```python
from build123d import *

# Parameters (mm, degrees)
F0_R     = 6.35
F1_DEPTH = 60
F3_DEPTH = 12
F4_R     = 1.5
F5_DEPTH = 25


with BuildPart() as f1:
    # F0 (on Front) → F1 (new body)
    with BuildSketch(Plane.XZ):
        Circle(F0_R)
    extrude(amount=-F1_DEPTH)

    # F2 (on face) → F3 (cut)
    with BuildSketch(Plane(origin=(0, 60, 0), x_dir=(-1, 0, 0), z_dir=(0, 1, 0))):
        Polygon((-6.955139, 0), (-4.5, -7.185974), (-4.5, 7.369376), align=None)
        Polygon((4.5, 7.369376), (4.5, -7.185974), (6.955139, 0), align=None)
    extrude(amount=-F3_DEPTH, mode=Mode.SUBTRACT)

    # F4 (on face) → F5 (cut)
    with BuildSketch(Plane.YZ.offset(4.5)):
        with Locations((56, 0)):
            Circle(F4_R)
    extrude(amount=-F5_DEPTH, mode=Mode.SUBTRACT)


solid = f1.part
```
Could you check a few things on this model? Use its own coordinates, in mm. A direction names the side the tool comes from. Round coordinates to 2 decimals unless told otherwise and drop trailing zeros. Loops run counter-clockwise (first coordinate to the right, second up) from the corner with the lowest first, then second, coordinate; pieces in that order, holes last. Notation, with made-up numbers: M 31,-25 L 88,-25 A19 cw 88,-21 Z; hole C -8.75,63.25 d7. An arc over 180 degrees is marked long. Answer as CSV lines item,"result".
1) We'd pull the mould along Z, two halves only. Please class faces 4 (the cylindrical face through (6.057, 29.58, 1.907)), 5 (the flat face through (4.5, 54, 0)), 6 (the cylindrical face through (0.06, 57.43, 0.45)): released by +Z, released by -Z, zero draft, split by the parting line, or undercut.
From the geometry:
face 4,"split by the parting line"
face 5,"zero draft"
face 6,"undercut"
2) Imagine slicing it at D-D on y = 24. List the corners of the cut face in (x, z) for me.
From the geometry:
outline,"C 0,0 d12.7"
3) Imagine slicing it at A-A on z = 0. List the corners of the cut face in (x, y) for me, and give its area (3 significant figures).
From the geometry:
outline,"M -6.35,0 L 6.35,0 L 6.35,48 L 4.5,48 L 4.5,54.5 L -4.5,54.5 L -4.5,48 L -6.35,48 Z; M -4.5,57.5 L 4.5,57.5 L 4.5,60 L -4.5,60 Z"
area,"691 mm^2"
4) Which directions (+Z, -Z, +X, -X, +Y, -Y) give clear straight access to the entire face, cutting with the end or side of a thin tool? Please do faces 1 (the flat face through (5, 48, 0)), 2 (the flat face through (0, 0, 0)), 3 (the flat face through (-4.5, 54, 0)).
From the geometry:
face 1,"+Z, -Z, +X, +Y"
face 2,"+Z, -Z, +X, -X, -Y"
face 3,"+Z, -Z, -X, +Y"
5) Imagine slicing it at C-C on x = 3.25. List the corners of the cut face in (y, z) for me, and give its area (3 significant figures).
From the geometry:
outline,"M 0,-5.46 L 60,-5.46 L 60,5.46 L 0,5.46 Z; hole C 56,0 d3"
area,"648 mm^2"
6) For pin 1 Ø0.6 at (x, z) = (5.5, 0.5) entering from +Y; pin 2 Ø3.5 at (y, z) = (56, 0) entering from -X; pin 3 Ø7 at (y, z) = (55, -1.5) entering from +X, each with a flat end and sliding along its axis, tell me the tip position at first contact or that it passes through.
From the geometry:
pin 1,"y = 48"
pin 2,"x = -4.5"
pin 3,"x = 4.5"
7) Imagine slicing it at B-B on y = 56. List the corners of the cut face in (x, z) for me.
From the geometry:
outline,"M -4.5,-4.48 A6.35 ccw 4.5,-4.48 L 4.5,-1.5 L -4.5,-1.5 Z; M -4.5,1.5 L 4.5,1.5 L 4.5,4.48 A6.35 ccw -4.5,4.48 Z"
8) If I drill on probe 1 along Z at (x, y) = (0, 56); probe 2 along X at (y, z) = (52, -3.75); probe 3 along Y at (x, z) = (5.25, -1.25), over which ranges is the centre line in solid material (lowest first)?
From the geometry:
probe 1,"-6.35 to -1.5, 1.5 to 6.35"
probe 2,"-4.5 to 4.5"
probe 3,"0 to 48"
